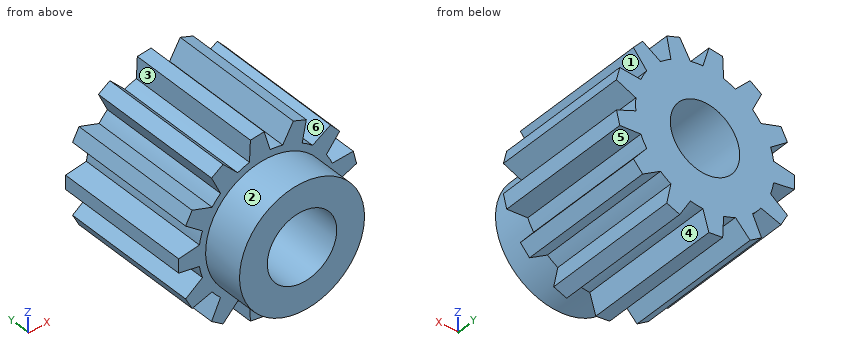
from build123d import *

# Parameters (mm, degrees)
SKETCH1_R           = 4.5
SKETCH1_R_2         = 2.5
BOSS_EXTRUDE1_DEPTH = 3
SKETCH2_R           = 5
SKETCH2_R_2         = 2.5
BOSS_EXTRUDE2_DEPTH = 10
BOSS_EXTRUDE3_DEPTH = 10


with BuildPart() as part:
    # Sketch1 → Boss-Extrude1 (new body)
    with BuildSketch(Plane(origin=(0, 0, 0), x_dir=(1, 0, 0), z_dir=(0, 1, 0))):
        with Locations(Location((0, 0, 0), (0, 0, 270))):
            Circle(SKETCH1_R)
        with Locations(Location((0, 0, 0), (0, 0, 270))):
            Circle(SKETCH1_R_2, mode=Mode.SUBTRACT)
    extrude(amount=BOSS_EXTRUDE1_DEPTH)

    # Sketch2 → Boss-Extrude2 (add)
    with BuildSketch(Plane(origin=(0, 3, 0), x_dir=(1, 0, 0), z_dir=(0, 1, 0))):
        with Locations(Location((0, 0, 0), (0, 0, 270))):
            Circle(SKETCH2_R)
        with Locations(Location((0, 0, 0), (0, 0, 270))):
            Circle(SKETCH2_R_2, mode=Mode.SUBTRACT)
    extrude(amount=BOSS_EXTRUDE2_DEPTH)

    # Sketch3 → Boss-Extrude3 (add)
    with BuildSketch(Plane(origin=(0, 13, 0), x_dir=(1, 0, 0), z_dir=(0, 1, 0))):
        Polygon((-4.943429983, -0.75), (-4.943429983, 0.75), (-6.443429983, 0.5), (-6.443429983, -0.5), align=None)
        Polygon((-5.473012319, 3.437139234), (-4.028647487, 2.961418482), (-4.725732245, 1.633234443), (-5.937735491, 2.551683208), align=None)
        Polygon((-3.248793489, 5.586871291), (-2.190950402, 4.494411678), (-3.425426201, 3.642314558), (-4.071777355, 5.018806544), align=None)
        Polygon((-0.280315223, 6.456718464), (0.148667016, 4.997789323), (-1.340396295, 4.816984303), (-1.273024097, 6.336181784), align=None)
        Polygon((2.752379883, 5.847409249), (2.454226613, 4.356233664), (1.051702249, 4.888140994), (1.81736364, 6.202014137), align=None)
        Polygon((5.154537927, 3.898529045), (4.197552469, 2.71671737), (3.202868482, 3.839483492), (4.491415268, 4.647039793), align=None)
        Polygon((6.375853451, 1.056542818), (4.979269641, 0.454833867), (4.620296144, 1.911246593), (6.136537786, 2.027484635), align=None)
        Polygon((6.136537786, -2.027484635), (4.620296144, -1.911246593), (4.979269641, -0.454833867), (6.375853451, -1.056542818), align=None)
        Polygon((4.491415268, -4.647039793), (3.202868482, -3.839483492), (4.197552469, -2.71671737), (5.154537927, -3.898529045), align=None)
        Polygon((1.81736364, -6.202014137), (1.051702249, -4.888140994), (2.454226613, -4.356233664), (2.752379883, -5.847409249), align=None)
        Polygon((-1.273024097, -6.336181784), (-1.340396295, -4.816984303), (0.148667016, -4.997789323), (-0.280315223, -6.456718464), align=None)
        Polygon((-4.071777355, -5.018806544), (-3.425426201, -3.642314558), (-2.190950402, -4.494411678), (-3.248793489, -5.586871291), align=None)
        Polygon((-5.937735491, -2.551683208), (-4.725732245, -1.633234443), (-4.028647487, -2.961418482), (-5.473012319, -3.437139234), align=None)
    extrude(amount=-BOSS_EXTRUDE3_DEPTH)


solid = part.part
The listing builds one solid part. Answer for the finished solid, in the listing's coordinates (mm). Face numbers are marked on the shaded views. A direction names the side the tool comes from. Give positions to 0.01 mm unless a question says otherwise; leave off trailing zeros. Order: outer loops, then holes, each group sorted by start corner. A loop starts at its lowest first (then second) coordinate and runs counter-clockwise, first axis right, second up. Notation, with made-up numbers: (-19, 35) - (4, 35) arc R18 cw to (4, 48) - close; hole circle Ø5 at (46.5, 11). An arc over 180 degrees is marked (long way). Use one line per item in the form item = value.
1) Find section A-A on z = 0. Determine the outline of the cut face in (x, y), and give its area (3 significant figures).
Verdict:
outline = (-6.44, 3) - (-4.5, 3) - (-4.5, 0) - (-2.5, 0) - (-2.5, 13) - (-6.44, 13) - close; (2.5, 0) - (4.5, 0) - (4.5, 3) - (5, 3) - (5, 13) - (2.5, 13) - close
area = 76.4 mm^2
2) Consider probe 1 along X at (y, z) = (10.5, 0); probe 2 along Z at (x, y) = (-3.5, 9); probe 3 along X at (y, z) = (2.5, 0). Determine where each line is inside the solid, lowest interval first. Write a range as [from, to].
Verdict:
probe_1 = [-6.44, -2.5], [2.5, 5]
probe_2 = [-5.41, -3.8], [-3.57, 3.57], [3.8, 5.41]
probe_3 = [-4.5, -2.5], [2.5, 4.5]
3) Find section C-C on x = 1.25. Determine the outline of the cut face in (y, z).
Verdict:
outline = (0, -4.32) - (3, -4.32) - (3, -5.23) - (13, -5.23) - (13, -2.17) - (0, -2.17) - close; (0, 2.17) - (13, 2.17) - (13, 5.23) - (3, 5.23) - (3, 4.32) - (0, 4.32) - close
4) Find section B-B on x = -3.75. Determine the outline of the cut face in (y, z), and give its area (3 significant figures).
Verdict:
outline = (0, -2.49) - (3, -2.49) - (3, -3.31) - (13, -3.31) - (13, 3.31) - (3, 3.31) - (3, 2.49) - (0, 2.49) - close; (3, -5.24) - (13, -5.24) - (13, -4.33) - (3, -4.33) - close; (3, 4.33) - (13, 4.33) - (13, 5.24) - (3, 5.24) - close
area = 99.2 mm^2
5) The mould has two halves that part along X. Classify the marked faces 1, 2 and 3: released by +X, released by -X, zero draft, split by the parting line, or undercut.
Verdict:
face_1 = released by +X
face_2 = split by the parting line
face_3 = undercut
6) For the marked faces 4, 5 and 6, determine the directions among +Z, -Z, +X, -X, +Y, -Y from which every point of the face is accessible in a straight line to the end or side of a thin tool.
Verdict:
face_4 = -Z, +Y, -Y
face_5 = +Y, -Y
face_6 = +Z, +Y, -Y
7) Each of these flat-tipped pins is pushed along its axis until it touches: pin 1 (4 mm diameter, centred on y = 6.5, z = 3, fed in from +X); pin 2 (3 mm diameter, centred on x = 1, y = 5.5, fed in from +Z); pin 3 (1 mm diameter, centred on y = 8, z = 4.5, fed in from +X); pin 4 (1 mm diameter, centred on x = -4, y = 5, fed in from +Z). Where does it stop, or does it pass through?
Verdict:
pin_1 = 6.38
pin_2 = 6.46
pin_3 = 5.06
pin_4 = 5.41
8) Find section D-D on x = 4. Determine the outline of the cut face in (y, z), and give its area (3 significant figures).
Verdict:
outline = (0, -2.06) - (3, -2.06) - (3, -4.34) - (13, -4.34) - (13, 4.34) - (3, 4.34) - (3, 2.06) - (0, 2.06) - close
area = 99.2 mm^2
